For this review, take the finished solid that the model builds, in its own axes (mm). A direction names the side the tool comes from. Coordinates: 2 decimals unless noted, no trailing zeros. Order: outer loops, then holes, each group sorted by start corner. A loop starts at its lowest first (then second) coordinate and runs counter-clockwise, first axis right, second up. Notation, with made-up numbers: (18.25, 3) -> (68.25, 3) arc R13 cw to (68.25, 20) -> close; hole circle Ø10 at (-2.5, -27.75). An arc over 180 degrees is marked (long way). Return JSON: item names as keys, results as strings. Group by question number.
Item 1: Take a section at C-C (z = -1.5). Write out the cut boundary in (x, y), then the cut area to 3 significant figures.
Item 2: For line 1 along Z through (x, y) = (-3, -3.5) (3 decimals); line 2 along Z through (x, y) = (-2.5, 18); line 3 along Y through (x, z) = (-2, 23), list the stretches that pass through material, from the lowest coordinate up.
Item 3: Machinability: for faces 4 (the cylindrical face through (-1.764, -3.391, -5.75)), 5 (the flat face through (4.94, 0, 19)), 6 (the flat face through (-5.004, 0, 7)), which of the approach directions +Z, -Z, +X, -X, +Y, -Y give a long, thin tool a straight path to every point of the face, cutting with its end or side? Answer none if there is none.
Item 4: Take a section at D-D (y = 11). Write out the cut boundary in (x, z).
Item 5: Insertion check: pin 1 (6 mm diameter, centred on x = -5.5, z = 27.5, fed in from -Y); pin 2 (1.8 mm diameter, centred on x = 0.5, z = 26, fed in from -Y); pin 3 (2 mm diameter, centred on x = 14.5, y = 3, fed in from -Z). Each pin has a flat end and moves straight along its axis. Give the tip position at first contact, or say it passes through.
Item 6: Draft analysis for pull direction Z (two halves, no side actions). For faces 1 (the cylindrical face through (2.837, 5.107, -1.565)), 2 (the flat face through (4, -5, 14.808)), 3 (the flat face through (-1, 0, -3.175)), state which applies: +Z half, -Z half, draft (parallel to the pull), parting line (faces both ways), or undercut.
Item 7: Take a section at A-A (x = 3). Write out the cut boundary in (y, z) (3 decimals), then the cut area to 3 significant figures.
```python
from build123d import *

# Parameters (mm, degrees)
BOSS_EXTRUDE1_DEPTH = 14.8082
SKETCH2_W           = 9.8806
SKETCH2_H           = 11.8618
BOSS_EXTRUDE2_DEPTH = 9.017
BOSS_EXTRUDE3_DEPTH = 9.9441
BOSS_EXTRUDE4_START = -6.4262
SKETCH4_R           = 20.0025
BOSS_EXTRUDE4_DEPTH = 6.4262
BOSS_EXTRUDE5_DEPTH = 3.175
SKETCH7_R           = 0.254
BOSS_EXTRUDE6_DEPTH = 1.4732
SKETCH8_R           = 3.8227
BOSS_EXTRUDE7_DEPTH = 2.2352


with BuildPart() as part:
    # Sketch1 → Boss-Extrude1 (new body)
    with BuildSketch(Plane.XY):
        with BuildLine():
            Line((-5.0038, 3.300729756), (-5.0038, -3.300729756))
            ThreePointArc((-5.0038, -3.300729756), (0, -5.9944), (5.0038, -3.300729756))
            Line((5.0038, -3.300729756), (5.0038, 3.300729756))
            ThreePointArc((5.0038, 3.300729756), (0, 5.9944), (-5.0038, 3.300729756))
        make_face()
    extrude(amount=BOSS_EXTRUDE1_DEPTH)

    # Sketch2 → Boss-Extrude2 (add)
    with BuildSketch(Plane.XY.offset(14.8082)):
        Rectangle(SKETCH2_W, SKETCH2_H)
    extrude(amount=BOSS_EXTRUDE2_DEPTH)

    # Sketch3 → Boss-Extrude3 (add)
    with BuildSketch(Plane.XY.offset(23.8252)):
        with BuildLine():
            Line((-1.112972237, -0.9652), (1.112972237, -0.9652))
            ThreePointArc((1.112972237, -0.9652), (0, 1.4732), (-1.112972237, -0.9652))
        make_face()
    extrude(amount=BOSS_EXTRUDE3_DEPTH)

    # Sketch4 → Boss-Extrude4 (add)
    with BuildSketch(Plane.XY.offset(33.7693).offset(BOSS_EXTRUDE4_START)):
        Circle(SKETCH4_R)
        with BuildLine():
            Line((-1.112972237, -0.9652), (1.112972237, -0.9652))
            ThreePointArc((1.112972237, -0.9652), (0, 1.4732), (-1.112972237, -0.9652))
        make_face(mode=Mode.SUBTRACT)
    extrude(amount=BOSS_EXTRUDE4_DEPTH)

    # Sketch5 → Boss-Extrude5 (add)
    with BuildSketch(Plane(origin=(0, 0, 0), x_dir=(-1, 0, 0), z_dir=(0, 0, -1))):
        with BuildLine():
            Line((0, -5.842), (5.4864, -5.842))
            Line((5.4864, -5.842), (5.4864, 5.842))
            Line((5.4864, 5.842), (0, 5.842))
            ThreePointArc((0, 5.842), (-2.873554597, 5.086417991), (-5.0038, 3.015120157))
            Line((-5.0038, 3.015120157), (-5.0038, -3.015120157))
            ThreePointArc((-5.0038, -3.015120157), (-2.873554597, -5.086417991), (0, -5.842))
        make_face()
    extrude(amount=BOSS_EXTRUDE5_DEPTH)

    # Sketch7 → Boss-Extrude6 (add)
    with BuildSketch(Plane(origin=(0, 0, -3.175), x_dir=(-1, 0, 0), z_dir=(0, 0, -1))):
        Circle(SKETCH7_R)
    extrude(amount=BOSS_EXTRUDE6_DEPTH)

    # Sketch8 → Boss-Extrude7 (add)
    with BuildSketch(Plane(origin=(0, 0, -4.6482), x_dir=(-1, 0, 0), z_dir=(0, 0, -1))):
        Circle(SKETCH8_R)
    extrude(amount=BOSS_EXTRUDE7_DEPTH)


solid = part.part
```
Findings below:
{
 "1": {"outline": "(-5.49, -5.84) -> (0, -5.84) arc R5.84 ccw to (5, -3.02) -> (5, 3.02) arc R5.84 ccw to (0, 5.84) -> (-5.49, 5.84) -> close", "area": "114 mm2"},
 "2": {"line 1": "z = -3.175 to 23.825, 27.343 to 33.769", "line 2": "z = 27.34 to 33.77", "line 3": "y = -5.93 to 5.93"},
 "3": {"face 4": "-Z", "face 5": "+X, +Y, -Y", "face 6": "-X, +Y, -Y"},
 "4": {"outline": "(-16.71, 27.34) -> (16.71, 27.34) -> (16.71, 33.77) -> (-16.71, 33.77) -> close"},
 "5": {"pin 1": "stops at y = -19.85", "pin 2": "stops at y = -0.97", "pin 3": "stops at z = 27.34"},
 "6": {"face 1": "draft", "face 2": "-Z half", "face 3": "undercut"},
 "7": {"outline": "(-19.776, 27.343) -> (19.776, 27.343) -> (19.776, 33.769) -> (-19.776, 33.769) -> close; (-5.931, 14.808) -> (-5.19, 14.808) -> (-5.19, 0) -> (-5.013, 0) -> (-5.013, -3.175) -> (5.013, -3.175) -> (5.013, 0) -> (5.19, 0) -> (5.19, 14.808) -> (5.931, 14.808) -> (5.931, 23.825) -> (-5.931, 23.825) -> close; (-2.369, -6.883) -> (2.369, -6.883) -> (2.369, -4.648) -> (-2.369, -4.648) -> close", "area": "557 mm2"}
}
